```python
from build123d import *

# Parameters (mm, degrees)
SKETCH_1_R          = 1.5
EXTRUDE_1_DEPTH     = 3
SKETCH_2_R          = 1.5
SKETCH_2_R_2        = 1.25
SKETCH_2_W          = 20
SKETCH_2_H          = 16
CUT_EXTRUDE_1_DEPTH = 31
SKETCH_3_W          = 24
SKETCH_3_H          = 6
SKETCH_3_W_2        = 6
SKETCH_3_H_2        = 18
CUT_EXTRUDE_2_DEPTH = 10
SKETCH_5_R          = 1.5
CUT_EXTRUDE_3_DEPTH = 10
CUT_EXTRUDE_4_DEPTH = 3


with BuildPart() as part:
    # 草图1 → 凸台-拉伸1 (new body)
    with BuildSketch(Plane(origin=(0, 0, 0), x_dir=(1, 0, 0), z_dir=(0, 1, 0))):
        with BuildLine():
            Line((-12.5, -50), (-12.5, -81))
            ThreePointArc((-12.5, -81), (-11.914213562, -82.414213562), (-10.5, -83))
            Line((-10.5, -83), (10.5, -83))
            ThreePointArc((10.5, -83), (11.914213562, -82.414213562), (12.5, -81))
            Line((12.5, -81), (12.5, -50))
            ThreePointArc((12.5, -50), (13.085786438, -48.585786438), (14.5, -48))
            Line((14.5, -48), (67.5, -48))
            Line((67.5, -48), (67.5, 48))
            Line((67.5, 48), (-67.5, 48))
            Line((-67.5, 48), (-67.5, -48))
            Line((-67.5, -48), (-14.5, -48))
            ThreePointArc((-14.5, -48), (-13.085786438, -48.585786438), (-12.5, -50))
        make_face()
        with Locations(Location((-37.123106012, 26.516504294, 0), (0, 0, 270))):
            Circle(SKETCH_1_R, mode=Mode.SUBTRACT)
        with Locations(Location((-26.516504294, 37.123106012, 0), (0, 0, 270))):
            Circle(SKETCH_1_R, mode=Mode.SUBTRACT)
        with Locations(Location((26.516504294, 37.123106012, 0), (0, 0, 90))):
            Circle(SKETCH_1_R, mode=Mode.SUBTRACT)
        with Locations(Location((37.123106012, 26.516504294, 0), (0, 0, 90))):
            Circle(SKETCH_1_R, mode=Mode.SUBTRACT)
        with Locations(Location((37.123106012, -26.516504294, 0), (0, 0, 270))):
            Circle(SKETCH_1_R, mode=Mode.SUBTRACT)
        with Locations(Location((26.516504294, -37.123106012, 0), (0, 0, 270))):
            Circle(SKETCH_1_R, mode=Mode.SUBTRACT)
        with Locations(Location((-37.123106012, -26.516504294, 0), (0, 0, 90))):
            Circle(SKETCH_1_R, mode=Mode.SUBTRACT)
        with Locations(Location((-26.516504294, -37.123106012, 0), (0, 0, 90))):
            Circle(SKETCH_1_R, mode=Mode.SUBTRACT)
    extrude(amount=EXTRUDE_1_DEPTH)

    # 草图2 → 切除-拉伸1 (cut)
    with BuildSketch(Plane(origin=(0, 3, 0), x_dir=(1, 0, 0), z_dir=(0, 1, 0))):
        with Locations(Location((-40, 13.5, 0), (0, 0, 270))):
            Circle(SKETCH_2_R)
        with Locations(Location((-40, -13.5, 0), (0, 0, 270))):
            Circle(SKETCH_2_R)
        with Locations(Location((-65, 13.5, 0), (0, 0, 270))):
            Circle(SKETCH_2_R)
        with Locations(Location((-65, -13.5, 0), (0, 0, 270))):
            Circle(SKETCH_2_R)
        with Locations(Location((40, -13.5, 0), (0, 0, 270))):
            Circle(SKETCH_2_R)
        with Locations(Location((40, 13.5, 0), (0, 0, 270))):
            Circle(SKETCH_2_R)
        with Locations(Location((65, -13.5, 0), (0, 0, 270))):
            Circle(SKETCH_2_R)
        with Locations(Location((65, 13.5, 0), (0, 0, 270))):
            Circle(SKETCH_2_R)
        with Locations(Location((-15.25, 27.25, 0), (0, 0, 270))):
            Circle(SKETCH_2_R_2)
        with Locations(Location((15.25, 27.25, 0), (0, 0, 270))):
            Circle(SKETCH_2_R_2)
        with Locations(Location((15.25, -3.25, 0), (0, 0, 270))):
            Circle(SKETCH_2_R_2)
        with Locations(Location((-15.25, -3.25, 0), (0, 0, 270))):
            Circle(SKETCH_2_R_2)
        with BuildLine():
            Line((4.25, -43), (4.25, -37))
            ThreePointArc((4.25, -37), (3, -35.75), (1.75, -37))
            Line((1.75, -37), (1.75, -43))
            ThreePointArc((1.75, -43), (3, -44.25), (4.25, -43))
        make_face()
        with BuildLine():
            Line((-4.25, -43), (-4.25, -37))
            ThreePointArc((-4.25, -37), (-3, -35.75), (-1.75, -37))
            Line((-1.75, -37), (-1.75, -43))
            ThreePointArc((-1.75, -43), (-3, -44.25), (-4.25, -43))
        make_face()
        with Locations((0, -16)):
            Rectangle(SKETCH_2_W, SKETCH_2_H)
    extrude(amount=-CUT_EXTRUDE_1_DEPTH, mode=Mode.SUBTRACT)

    # 草图3 → 切除-拉伸2 (cut)
    with BuildSketch(Plane(origin=(0, 3, 0), x_dir=(1, 0, 0), z_dir=(0, 1, 0))):
        with Locations((0, 40)):
            Rectangle(SKETCH_3_W, SKETCH_3_H)
        with Locations((31, 0)):
            Rectangle(SKETCH_3_W_2, SKETCH_3_H_2)
        with Locations((-31, 0)):
            Rectangle(SKETCH_3_W_2, SKETCH_3_H_2)
    extrude(amount=-CUT_EXTRUDE_2_DEPTH, mode=Mode.SUBTRACT)

    # 草图5 → 切除-拉伸3 (cut)
    with BuildSketch(Plane(origin=(0, 3, 0), x_dir=(1, 0, 0), z_dir=(0, 1, 0))):
        with Locations(Location((-64.5, 30, 0), (0, 0, 270))):
            Circle(SKETCH_5_R)
        with Locations(Location((64.5, 30, 0), (0, 0, 270))):
            Circle(SKETCH_5_R)
        with Locations(Location((64.5, -30, 0), (0, 0, 270))):
            Circle(SKETCH_5_R)
        with Locations(Location((-64.5, -30, 0), (0, 0, 270))):
            Circle(SKETCH_5_R)
        with BuildLine():
            Line((-24.468037432, 46.242640687), (-44.780190541, 25.930487577))
            ThreePointArc((-44.780190541, 25.930487577), (-54.578308632, 23.380578475), (-61.58105962, 30.692666628))
            ThreePointArc((-61.58105962, 30.692666628), (-64.848696759, 32.979666184), (-67.5, 30))
            Line((-67.5, 30), (-67.5, 48))
            Line((-67.5, 48), (-20.225396744, 48))
            ThreePointArc((-20.225396744, 48), (-22.521497339, 47.543277195), (-24.468037432, 46.242640687))
        make_face()
        with BuildLine():
            Line((67.5, 48), (67.5, 30))
            ThreePointArc((67.5, 30), (64.848696759, 32.979666184), (61.58105962, 30.692666628))
            ThreePointArc((61.58105962, 30.692666628), (54.578308632, 23.380578475), (44.780190541, 25.930487577))
            Line((44.780190541, 25.930487577), (24.468037432, 46.242640687))
            ThreePointArc((24.468037432, 46.242640687), (22.521497339, 47.543277195), (20.225396744, 48))
            Line((20.225396744, 48), (67.5, 48))
        make_face()
        with BuildLine():
            Line((67.5, -48), (67.5, -30))
            ThreePointArc((67.5, -30), (64.848696759, -32.979666184), (61.58105962, -30.692666628))
            ThreePointArc((61.58105962, -30.692666628), (54.578308632, -23.380578475), (44.780190541, -25.930487577))
            Line((44.780190541, -25.930487577), (24.468037432, -46.242640687))
            ThreePointArc((24.468037432, -46.242640687), (22.521497339, -47.543277195), (20.225396744, -48))
            Line((20.225396744, -48), (67.5, -48))
        make_face()
        with BuildLine():
            Line((-20.225396744, -48), (-67.5, -48))
            Line((-67.5, -48), (-67.5, -30))
            ThreePointArc((-67.5, -30), (-64.848696759, -32.979666184), (-61.58105962, -30.692666628))
            ThreePointArc((-61.58105962, -30.692666628), (-54.578308632, -23.380578475), (-44.780190541, -25.930487577))
            Line((-44.780190541, -25.930487577), (-24.468037432, -46.242640687))
            ThreePointArc((-24.468037432, -46.242640687), (-22.521497339, -47.543277195), (-20.225396744, -48))
        make_face()
    extrude(amount=-CUT_EXTRUDE_3_DEPTH, mode=Mode.SUBTRACT)

    # 草图6 → 切除-拉伸4 (cut)
    with BuildSketch(Plane(origin=(0, 3, 0), x_dir=(1, 0, 0), z_dir=(0, 1, 0))):
        with BuildLine():
            Line((-10, 46), (10, 46))
            ThreePointArc((10, 46), (12.547371205, 46.246783902), (15, 46.977957164))
            ThreePointArc((15, 46.977957164), (17.563191705, 47.742091241), (20.225396744, 48))
            Line((20.225396744, 48), (20.225396744, 49))
            Line((20.225396744, 49), (-20.225396744, 49))
            Line((-20.225396744, 49), (-20.225396744, 48))
            ThreePointArc((-20.225396744, 48), (-17.563191705, 47.742091241), (-15, 46.977957164))
            ThreePointArc((-15, 46.977957164), (-12.547371205, 46.246783902), (-10, 46))
        make_face()
        with BuildLine():
            Line((-4.371087012, -81.471994656), (-12.5, -48))
            ThreePointArc((-12.5, -48), (-17.891385365, -43.085345419), (-24.468037432, -46.242640687))
            Line((-24.468037432, -46.242640687), (-24.468037432, -84))
            Line((-24.468037432, -84), (24.468037432, -84))
            Line((24.468037432, -84), (24.468037432, -46.242640687))
            ThreePointArc((24.468037432, -46.242640687), (17.891385365, -43.085345419), (12.5, -48))
            Line((12.5, -48), (4.371087012, -81.471994656))
            ThreePointArc((4.371087012, -81.471994656), (3.663704737, -82.572257821), (2.427579604, -83))
            Line((2.427579604, -83), (-2.427579604, -83))
            ThreePointArc((-2.427579604, -83), (-3.663704737, -82.572257821), (-4.371087012, -81.471994656))
        make_face()
    extrude(amount=-CUT_EXTRUDE_4_DEPTH, mode=Mode.SUBTRACT)


solid = part.part
```
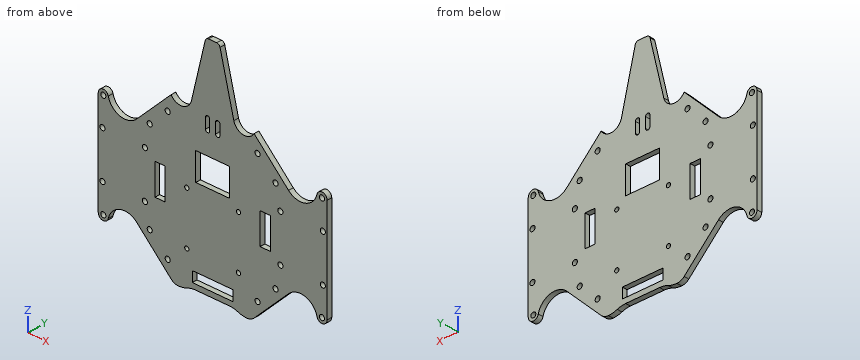
The model under review builds one solid part; all positions refer to its coordinate system, in mm. Give positions to 0.01 mm unless a question says otherwise; leave off trailing zeros. Order: outer loops, then holes, each group sorted by start corner. A loop starts at its lowest first (then second) coordinate and runs counter-clockwise, first axis right, second up. Notation, with made-up numbers: (0, 28) - (44, 28) arc R20 cw to (44, 33) - close; hole circle Ø2 at (-16.5, 21). An arc over 180 degrees is marked (long way). Use CSV: the item, a comma, the result in double quotes. Start each with the question number.
Q1. To check wall thickness, follow line 1 along X through (y, z) = (0.75, 0); line 2 along X through (y, z) = (1.05, 3.25); line 3 along X through (y, z) = (1.4, 15.5). State the ranges of each line that lie inside material, in increasing order. Write a range as [from, to].
Q2. We need section C-C, the plane x = -55.5. Write out the cut boundary in (y, z), and give its area (3 significant figures).
Q3. We need section A-A, the plane z = 61. Write out the cut boundary in (x, y), and give its area (3 significant figures).
Q4. We need section B-B, the plane y = 1.75. State how many separate pieces and enclosed holes the cut face has, and give its area (3 significant figures).
Q5. Clearance check with a flat-ended pin moving along its axis: pin 1 Ø2.5 at (x, z) = (65, -13.5) entering from +Y. State where the tip first meets the part, or that it passes through.
Outcome:
1,line 1,"x = [-67.5, -34], [-28, 28], [34, 67.5]"
1,line 2,"x = [-67.5, -34], [-28, -16.5], [-14, 14], [16.5, 28], [34, 67.5]"
1,line 3,"x = [-67.5, -10], [10, 67.5]"
2,outline,"(0, -23.69) - (3, -23.69) - (3, 23.69) - (0, 23.69) - close"
2,area,"142 mm^2"
3,outline,"(-9.34, 0) - (9.34, 0) - (9.34, 3) - (-9.34, 3) - close"
3,area,"56.1 mm^2"
4,separate pieces,"1"
4,enclosed holes,"30"
4,area,"9,580 mm^2"
5,pin 1,"passes through"
